```python
from build123d import *

# Parameters (mm, degrees)
F0_W     = 25.4
F0_H     = 25.4
F1_DEPTH = 50.8
F2_W     = 4.558041
F2_H     = 25.4
F3_DEPTH = 12.7
F4_W     = 11.245678
F4_H     = 21.608493
F5_DEPTH = 25.4


with BuildPart() as f1:
    # F0 (on Front) → F1 (new body)
    with BuildSketch(Plane.XZ):
        with Locations((-21.452703, 12.7)):
            Rectangle(F0_W, F0_H)
    extrude(amount=F1_DEPTH)

    # F2 (on face) → F3 (join)
    with BuildSketch(Plane(origin=(-34.152703, 0, 0), x_dir=(0, -1, 0), z_dir=(-1, 0, 0))):
        with Locations((24.176082, 12.7)):
            Rectangle(F2_W, F2_H)
    extrude(amount=F3_DEPTH)

    # F4 (on face) → F5 (cut)
    with BuildSketch(Plane(origin=(0, -21.897061, 0), x_dir=(-1, 0, 0), z_dir=(0, 1, 0))):
        with Locations((39.775542, 12.82661)):
            Rectangle(F4_W, F4_H)
    extrude(amount=-F5_DEPTH, mode=Mode.SUBTRACT)


solid = f1.part
```
Work out the finished part from the listing and answer in its coordinate system (mm). A direction names the side the tool comes from. Round coordinates to 2 decimals unless told otherwise and drop trailing zeros. Write each loop counter-clockwise with the first axis right and the second up, starting at its lowest first coordinate (ties: lowest second). Pieces come first, ordered by that corner, then holes. Notation, with made-up numbers: (3, 6.5) -> (58, 6.5) arc R26 cw to (58, 25.5) -> close; hole circle Ø8 at (-19.75, 85). An arc over 180 degrees is marked (long way). Write each question's results on one line, items separated by ' | '.
1) Which of the six approach directions +Z, -Z, +X, -X, +Y, -Y give full straight-line access (tool end or side, diameter ignored) to faces 1 (the flat face through (-46, -21.897, 14)), 2 (the flat face through (-46, -26.455, 14)), 3 (the flat face through (-40, -24, 2.022)), 4 (the flat face through (-22, -50.8, 13)), 5 (the flat face through (-46.853, -24, 13))?
Findings:
face 1: +Z, -Z, -X, +Y | face 2: +Z, -Z, -X, -Y | face 3: +Y, -Y | face 4: +Z, -Z, +X, -X, -Y | face 5: +Z, -Z, -X, +Y, -Y
2) For a pull along X with two mould halves and no side action, classify faces 6 (the flat face through (-22, 0, 13)), 7 (the flat face through (-8.753, -25, 13)), 8 (the flat face through (-45.398, -24, 13)) as +X half, -X half, draft (parallel to the pull), parting line (faces both ways), or undercut.
Findings:
face 6: draft | face 7: +X half | face 8: undercut
3) Consider line 1 along X through (y, z) = (-26, 12); line 2 along Z through (x, y) = (-34.5, -22.5); line 3 along X through (y, z) = (-13, 14.5). Determine where each line is inside the solid, lowest interval first. Write a range as [from, to].
Findings:
line 1: x = [-46.85, -45.4], [-34.15, -8.75] | line 2: z = [0, 2.02], [23.63, 25.4] | line 3: x = [-34.15, -8.75]
4) Flat-ended cylindrical pins translate along their axes: pin 1 (10 mm diameter, centred on x = -40, z = 10.5, fed in from +Y); pin 2 (10 mm diameter, centred on x = -42, z = 17.5, fed in from +Y). Find the tip coordinate at first contact, or state that the pin passes through.
Findings:
pin 1: passes through | pin 2: stops at y = -21.9
5) The part is cut by section B-B (z = 4). Write down the section's boundary in (x, y), and give its area (3 significant figures).
Findings:
outline: (-46.85, -26.46) -> (-45.4, -26.46) -> (-45.4, -21.9) -> (-46.85, -21.9) -> close; (-34.15, -50.8) -> (-8.75, -50.8) -> (-8.75, 0) -> (-34.15, 0) -> close | area: 1,300 mm²
6) The part is cut by section A-A (x = -43.5). Write down the section's boundary in (y, z), and give its area (3 significant figures).
Findings:
outline: (-26.46, 0) -> (-21.9, 0) -> (-21.9, 2.02) -> (-26.46, 2.02) -> close; (-26.46, 23.63) -> (-21.9, 23.63) -> (-21.9, 25.4) -> (-26.46, 25.4) -> close | area: 17.3 mm²
7) The part is cut by section C-C (y = -45.5). Write down the section's boundary in (x, z).
Findings:
outline: (-34.15, 0) -> (-8.75, 0) -> (-8.75, 25.4) -> (-34.15, 25.4) -> close
